```python
from build123d import *

# Parameters (mm, degrees)
SKETCH1_R           = 25
BOSS_EXTRUDE1_DEPTH = 45
SKETCH2_R           = 24
BOSS_EXTRUDE2_DEPTH = 48
SKETCH3_R           = 2
BOSS_EXTRUDE3_DEPTH = 63


with BuildPart() as part:
    # Sketch1 → Boss-Extrude1 (new body)
    with BuildSketch(Plane.XY):
        Circle(SKETCH1_R)
    extrude(amount=BOSS_EXTRUDE1_DEPTH)

    # Sketch2 → Boss-Extrude2 (add)
    with BuildSketch(Plane.XY):
        Circle(SKETCH2_R)
    extrude(amount=BOSS_EXTRUDE2_DEPTH)

    # Sketch3 → Boss-Extrude3 (add)
    with BuildSketch(Plane.XY):
        Circle(SKETCH3_R)
    extrude(amount=BOSS_EXTRUDE3_DEPTH)


solid = part.part
```
Geometry check sheet. Reference: the model listing, model coordinates, mm. A direction names the side the tool comes from. Give positions to 0.01 mm unless a question says otherwise; leave off trailing zeros. Write each loop counter-clockwise with the first axis right and the second up, starting at its lowest first coordinate (ties: lowest second). Pieces come first, ordered by that corner, then holes. Notation, with made-up numbers: (-31, 23.5) -> (-25, 23.5) arc R19 cw to (-25, 33.5) -> close; hole circle Ø7 at (81, 40.5). An arc over 180 degrees is marked (long way). One line per question, with ' | ' between items.
Item 1: Access from +Z, -Z, +X, -X, +Y, -Y to the whole of each face (thin tool, end or side, straight path). Record for faces 1 (the flat face through (0, 0, 63)), 2 (the cylindrical face through (0, -2, 55)).
Determined:
face 1: +Z, +X, -X, +Y, -Y | face 2: +Z
Item 2: Sectioned sample at D-D, the plane y = -9. Record the boundary of the cut face in (x, z), plus the area to 3 significant figures.
Determined:
outline: (-23.32, 0) -> (23.32, 0) -> (23.32, 45) -> (22.25, 45) -> (22.25, 48) -> (-22.25, 48) -> (-22.25, 45) -> (-23.32, 45) -> close | area: 2,230 mm^2
Item 3: Depth check by flat-ended pin: pin 1 (6 mm diameter, centred on x = -19, y = 0, fed in from +Z); pin 2 (1 mm diameter, centred on y = 12.5, z = 26, fed in from -X); pin 3 (3 mm diameter, centred on y = 10.5, z = 26, fed in from +X). Enter the tip coordinate at first touch or a pass-through.
Determined:
pin 1: z = 48 | pin 2: x = -21.93 | pin 3: x = 23.32
Item 4: Sectioned sample at A-A, the plane y = 0. Record the boundary of the cut face in (x, z).
Determined:
outline: (-25, 0) -> (25, 0) -> (25, 45) -> (24, 45) -> (24, 48) -> (2, 48) -> (2, 63) -> (-2, 63) -> (-2, 48) -> (-24, 48) -> (-24, 45) -> (-25, 45) -> close
Item 5: Scan lines: line 1 along Z through (x, y) = (-13, 8); line 2 along Z through (x, y) = (15, 19.5); line 3 along Y through (x, z) = (10.5, 47). Record each from-to range of solid material in increasing order.
Determined:
line 1: 0 to 48 | line 2: 0 to 45 | line 3: -21.58 to 21.58
Item 6: Sectioned sample at C-C, the plane z = 13. Record the boundary of the cut face in (x, y), plus the area to 3 significant figures.
Determined:
outline: circle Ø50 at (0, 0) | area: 1,960 mm^2
